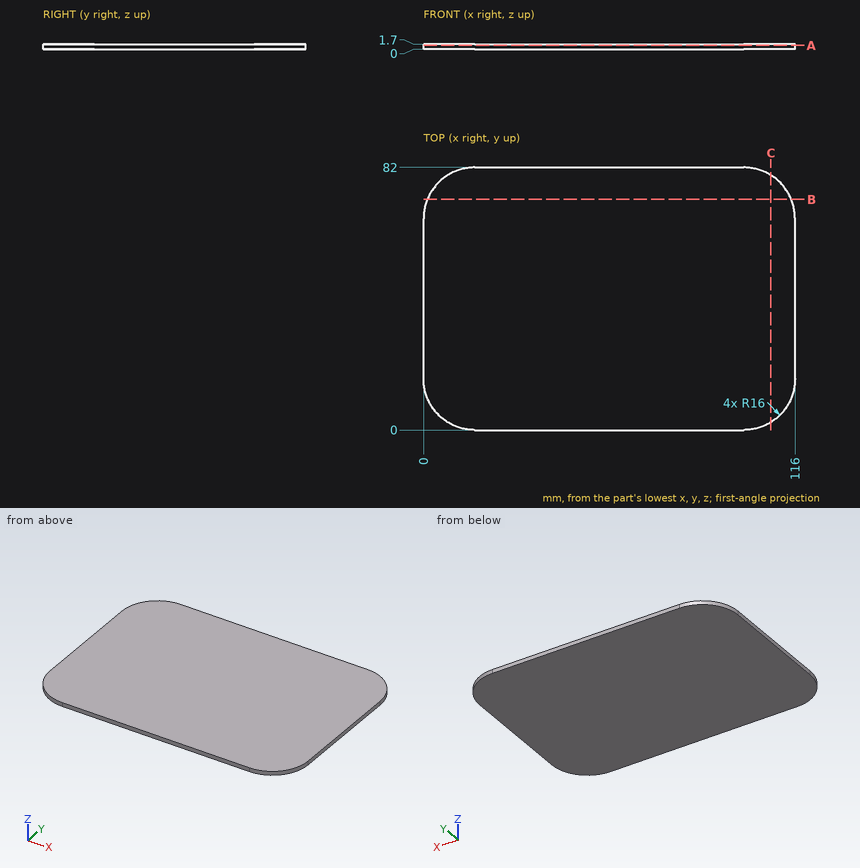
Verification items for this drawing (mm, ordinates from the low corner). Coordinates: 2 decimals unless noted, no trailing zeros. Write each loop counter-clockwise with the first axis right and the second up, starting at its lowest first coordinate (ties: lowest second). Pieces come first, ordered by that corner, then holes. Notation, with made-up numbers: M 17.5,78.5 L 39.5,78.5 A23 ccw 39.5,115.5 Z; hole C -23.5,-38 d9. An arc over 180 degrees is marked long. Answer as CSV lines item,"result".
Q1. Material ranges on probe 1 along X at (y, z) = (68, 1.1); probe 2 along X at (y, z) = (76, 1.45); probe 3 along Y at (x, z) = (104.5, 1.35), recorded low to high. Write a range as from..to.
Check result:
probe 1,"0.13..115.87"
probe 2,"3.51..112.49"
probe 3,"0.65..81.35"
Q2. Cross-section at C-C (x = 108.5). Record the boundary of the cut face in (y, z), then the cut area to 3 significant figures.
Check result:
outline,"M 2.44,0 L 79.56,0 L 79.56,1.7 L 2.44,1.7 Z"
area,"131 mm^2"
Q3. Go/stop test with a flat-tipped pin: pin 1 (10 mm diameter, centred on x = 64.5, y = 66.5, fed in from -Z). Record where the tip stops, or that it passes through.
Check result:
pin 1,"z = 0"
Q4. Cross-section at B-B (y = 72). Record the boundary of the cut face in (x, z), then the cut area to 3 significant figures.
Check result:
outline,"M 1.17,0 L 114.83,0 L 114.83,1.7 L 1.17,1.7 Z"
area,"193 mm^2"
Q5. Cross-section at A-A (z = 1.3). Record the boundary of the cut face in (x, y), then the cut area to 3 significant figures.
Check result:
outline,"M 0,16 A16 ccw 16,0 L 100,0 A16 ccw 116,16 L 116,66 A16 ccw 100,82 L 16,82 A16 ccw 0,66 Z"
area,"9,290 mm^2"
